Autodesk Inventor part; units mm, degrees
ref_plane "YZ Plane" through (0, 0, 0) normal (1, 0, 0) x (0, 1, 0)
ref_plane "XZ Plane" through (0, 0, 0) normal (0, 1, 0) x (-1, 0, 0)
ref_plane "XY Plane" through (0, 0, 0) normal (0, 0, 1) x (1, 0, 0)
sketch "Sketch1" plane through (0, 0, 0) normal (0, 0, 1) x (1, 0, 0)
  circle A0 centre (0, 0) radius 15.875
  circle A1 centre (0, 0) radius 23.8125 construction
  circle A2 centre (0, 23.8125) radius 2.2479
  circle A3 centre (-20.6222, 11.9063) radius 2.2479
  circle A4 centre (-20.6222, -11.9062) radius 2.2479
  circle A5 centre (0, -23.8125) radius 2.2479
  circle A6 centre (20.6222, -11.9063) radius 2.2479
  circle A7 centre (20.6222, 11.9062) radius 2.2479
  circle A8 centre (0, 0) radius 28.575
  dimension "d1" = 47.625
  dimension "d0" = 31.75
  dimension "d2" = 4.4958
  dimension "d5" = 360
  dimension "d7" = 57.15
extrude "Extrusion1" add sketch "Sketch1" along normal blind 38.1
properties part number "Spacer Between Wheels V2" material "Polycarbonate, Clear"
Geometry check sheet. Reference: the model listing, model coordinates, mm. Give positions to 0.01 mm unless a question says otherwise; leave off trailing zeros. Write each loop counter-clockwise with the first axis right and the second up, starting at its lowest first coordinate (ties: lowest second). Pieces come first, ordered by that corner, then holes.
1) Section check B-B, the plane y = 0. Record the boundary of the cut face in (x, z) (3 decimals).
2) Section check D-D, the plane z = 22.5. State how many separate pieces and enclosed holes the cut face has, and give its area (3 significant figures).
3) Release check for a two-part mould opening along Y. For faces 1 (the cylindrical face through (-0.487, 26.007, 18.783)), 2 (the cylindrical face through (-28.547, -1.256, 18.783)), 3 (the flat face through (12, -12, 0)) record: pulls with the +Y half, pulls with the -Y half, needs draft (parallel to the pull), parting line crosses it, or undercut.
4) Material ranges on L1, parallel to Y at x = 0, z = 13 (3 decimals); L2, parallel to Y at x = -21.5, z = 36; L3, parallel to Y at x = 1, z = 31, recorded low to high.
5) Section check A-A, the plane x = 0. Record the boundary of the cut face in (y, z) (3 decimals).
6) Gauge pin test, flat ends, axial feed: pin 1 (5 mm diameter, centred on x = -20.62, y = -11.91, fed in from -Z); pin 2 (2.5 mm diameter, centred on x = 20.62, y = 11.91, fed in from +Z); pin 3 (12 mm diameter, centred on x = 22.5, z = 33, fed in from +Y); pin 4 (8 mm diameter, centred on x = -7.5, z = 31, fed in from -Y). Record the tip position at first contact, or that the pin passes through.
7) Section check C-C, the plane x = 8.5. Record the boundary of the cut face in (y, z), and give its area (3 significant figures).
Computed:
1. outline: (-28.575, 0) - (-15.875, 0) - (-15.875, 38.1) - (-28.575, 38.1) - close; (15.875, 0) - (28.575, 0) - (28.575, 38.1) - (15.875, 38.1) - close
2. separate pieces: 1
2. enclosed holes: 7
2. area: 1,680 mm2
3. face 1: undercut
3. face 2: parting line crosses it
3. face 3: needs draft
4. L1: y = -28.575 to -26.06, -21.565 to -15.875, 15.875 to 21.565, 26.06 to 28.575
4. L2: y = -18.82 to -13.98, -9.84 to 9.84, 13.98 to 18.82
4. L3: y = -28.56 to -25.83, -21.8 to -15.84, 15.84 to 21.8, 25.83 to 28.56
5. outline: (-28.575, 0) - (-26.06, 0) - (-26.06, 38.1) - (-28.575, 38.1) - close; (-21.565, 0) - (-15.875, 0) - (-15.875, 38.1) - (-21.565, 38.1) - close; (15.875, 0) - (21.565, 0) - (21.565, 38.1) - (15.875, 38.1) - close; (26.06, 0) - (28.575, 0) - (28.575, 38.1) - (26.06, 38.1) - close
6. pin 1: stops at z = 0
6. pin 2: passes through
6. pin 3: stops at y = 23.33
6. pin 4: stops at y = -28.36
7. outline: (-27.28, 0) - (-13.41, 0) - (-13.41, 38.1) - (-27.28, 38.1) - close; (13.41, 0) - (27.28, 0) - (27.28, 38.1) - (13.41, 38.1) - close
7. area: 1,060 mm2
